from build123d import *

# Parameters (mm, degrees)
SKETCH1_W           = 19.05
SKETCH1_H           = 19.05
SKETCH1_R           = 1.5875
SKETCH1_R_2         = 3.96875
BOSS_EXTRUDE1_DEPTH = 2.54
SKETCH2_R           = 5.715
SKETCH2_R_2         = 4.92125
BOSS_EXTRUDE2_DEPTH = 9.525
FILLET1_R           = 0.79375
FILLET2_R           = 3.175


with BuildPart() as part:
    # Sketch1 → Boss-Extrude1 (new body)
    with BuildSketch(Plane(origin=(0, 0, 0), x_dir=(1, 0, 0), z_dir=(0, 1, 0))):
        Rectangle(SKETCH1_W, SKETCH1_H)
        with Locations(Location((-6.35, 6.35, 0), (0, 0, 270))):
            Circle(SKETCH1_R, mode=Mode.SUBTRACT)
        with Locations(Location((6.35, 6.35, 0), (0, 0, 270))):
            Circle(SKETCH1_R, mode=Mode.SUBTRACT)
        with Locations(Location((6.35, -6.35, 0), (0, 0, 270))):
            Circle(SKETCH1_R, mode=Mode.SUBTRACT)
        with Locations(Location((-6.35, -6.35, 0), (0, 0, 270))):
            Circle(SKETCH1_R, mode=Mode.SUBTRACT)
        with Locations(Location((0, 0, 0), (0, 0, 270))):
            Circle(SKETCH1_R_2, mode=Mode.SUBTRACT)
    extrude(amount=BOSS_EXTRUDE1_DEPTH)

    # Sketch2 → Boss-Extrude2 (add)
    with BuildSketch(Plane(origin=(0, 2.54, 0), x_dir=(1, 0, 0), z_dir=(0, 1, 0))):
        with Locations(Location((0, 0, 0), (0, 0, 90))):
            Circle(SKETCH2_R)
        with Locations(Location((0, 0, 0), (0, 0, 90))):
            Circle(SKETCH2_R_2, mode=Mode.SUBTRACT)
    extrude(amount=BOSS_EXTRUDE2_DEPTH)

    # Fillet1
    fillet1_edges = [part.edges().sort_by_distance(p)[0] for p in [
        (0, 2.54, 5.715),
        (0, 2.54, 4.92125),
    ]]
    fillet(fillet1_edges, radius=FILLET1_R)

    # Fillet2
    fillet2_edges = [part.edges().sort_by_distance(p)[0] for p in [
        (9.525, 1.27, 9.525),
        (-9.525, 1.27, 9.525),
        (-9.525, 1.27, -9.525),
        (9.525, 1.27, -9.525),
    ]]
    fillet(fillet2_edges, radius=FILLET2_R)


solid = part.part
Could you check a few things on this model? Use its own coordinates, in mm. A direction names the side the tool comes from. Give positions to 0.01 mm unless a question says otherwise; leave off trailing zeros. Order: outer loops, then holes, each group sorted by start corner. A loop starts at its lowest first (then second) coordinate and runs counter-clockwise, first axis right, second up.
1. For pin 1 (5 mm diameter, centred on x = 4.5, z = 5.5, fed in from -Y); pin 2 (4 mm diameter, centred on x = -1, z = 0.5, fed in from +Y); pin 3 (6 mm diameter, centred on x = 0.5, y = 6, fed in from +Z); pin 4 (1 mm diameter, centred on y = 5.5, z = -5.5, fed in from -X), each with a flat end and sliding along its axis, tell me the tip position at first contact or that it passes through.
Answers below:
pin 1: stops at y = 0
pin 2: passes through
pin 3: stops at z = 5.78
pin 4: stops at x = -2.77
2. Which directions (+Z, -Z, +X, -X, +Y, -Y) give clear straight access to the entire face, cutting with the end or side of a thin tool? Please do faces 4 (the cylindrical face through (-7.76, 1.25, -5.62)), 5 (the cylindrical face through (-5.666, 7.638, 0.744)).
Answers below:
face 4: +Y, -Y
face 5: +Y
3. I need wall thicknesses on L1, parallel to X at y = 1.55, z = -6.35 (1 decimal); L2, parallel to X at y = 1.6, z = 0 (3 decimals); L3, parallel to Z at x = 1, y = 2.75. Which ranges of each line are inside material? Lowest first, please.
Answers below:
L1: x = -9.5 to -7.9, -4.8 to 4.8, 7.9 to 9.5
L2: x = -9.525 to -3.969, 3.969 to 9.525
L3: z = -5.89 to -4.56, 4.56 to 5.89
4. Suppose I cut it at C-C (z = -6). State how many separate pieces and enclosed holes the cut face has, plus the area to 3 significant figures.
Answers below:
separate pieces: 3
enclosed holes: 0
area: 33.1 mm2
5. Suppose I cut it at B-B (y = 10.75). Write out the boundary of the cut face in (x, z) (1 decimal).
Answers below:
outline: circle Ø11.4 at (0, 0); hole circle Ø9.8 at (0, 0)
6. Thinking about a two-plate mould opening in X: for faces 1 (the flat face through (9.525, 1, 0)), 2 (the cylindrical face through (4.94, 1.25, -5.62)), 3 (the flat face through (0, 1, 9.525)), which applies, +X half, -X half, draft (parallel to the pull), parting line (faces both ways), or undercut?
Answers below:
face 1: +X half
face 2: undercut
face 3: draft
